Design review of the part built by this model. Coordinates are the model's own, in mm. A direction names the side the tool comes from. Give positions to 0.01 mm unless a question says otherwise; leave off trailing zeros. Loops run counter-clockwise (first coordinate to the right, second up) from the corner with the lowest first, then second, coordinate; pieces in that order, holes last. Notation, with made-up numbers: M 1.25,4.5 L 41.25,4.5 A29 cw 41.25,34.5 Z; hole C 47.5,38 d10. An arc over 180 degrees is marked long. Answer as CSV lines item,"result".
```python
from build123d import *

# Parameters (mm, degrees)
BOSS_EXTRUDE1_DEPTH = 8


with BuildPart() as part:
    # Sketch1 → Boss-Extrude1 (new body)
    with BuildSketch(Plane.XY):
        with BuildLine():
            Line((79.487889635, 127.207214423), (0, 0))
            Line((0, 0), (38, 0))
            ThreePointArc((38, 0), (40.636038969, 6.363961031), (47, 9))
            Line((47, 9), (99, 9))
            ThreePointArc((99, 9), (105.363961031, 6.363961031), (108, 0))
            Line((108, 0), (142, 0))
            Line((142, 0), (172.50354814, 93.880267937))
            ThreePointArc((172.50354814, 93.880267937), (166.569139078, 124.354715336), (137.573015724, 135.451290736))
            Line((137.573015724, 135.451290736), (79.487889635, 127.207214423))
        make_face()
        with BuildLine():
            ThreePointArc((130.852326035, 79.986711388), (131.785075785, 80.179945877), (132.735423682, 80.244757424))
            ThreePointArc((132.735423682, 80.244757424), (139.670612135, 74.195105322), (134.61852133, 66.50280346))
            ThreePointArc((134.61852133, 66.50280346), (133.68577158, 66.309568971), (132.735423682, 66.244757424))
            Line((132.735423682, 66.244757424), (99.049026675, 61.628618036))
            ThreePointArc((99.049026675, 61.628618036), (95.608426443, 60.298814317), (93.130184546, 57.566704329))
            ThreePointArc((93.130184546, 57.566704329), (61.402056741, 63.469750476), (90.372565984, 77.690497362))
            ThreePointArc((90.372565984, 77.690497362), (93.494426366, 75.725784751), (97.165929028, 75.370572))
            Line((97.165929028, 75.370572), (130.852326035, 79.986711388))
        make_face(mode=Mode.SUBTRACT)
    extrude(amount=BOSS_EXTRUDE1_DEPTH)


solid = part.part
```
1. We need section D-D, the plane x = 155. Write out the cut boundary in (y, z).
Answer block:
outline,"M 40.01,0 L 133.04,0 L 133.04,8 L 40.01,8 Z"
2. We need section C-C, the plane x = 68. Write out the cut boundary in (y, z).
Answer block:
outline,"M 9,0 L 52.21,0 L 52.21,8 L 9,8 Z; M 79.34,0 L 108.82,0 L 108.82,8 L 79.34,8 Z"
3. We need section B-B, the plane y = 52. Write out the cut boundary in (x, z), plus the area to 3 significant figures.
Answer block:
outline,"M 32.49,0 L 68.29,0 L 68.29,8 L 32.49,8 Z; M 88.2,0 L 158.9,0 L 158.9,8 L 88.2,8 Z"
area,"852 mm²"
4. For P1, Ø2, axis at y = 51, z = 2.5, coming from the +X side; P2, Ø1.5, axis at y = 19, z = 2, coming from the +X side; P3, Ø2, axis at y = 119.5, z = 4.5, coming from the +X side, all flat-tipped, find the tip position at first contact; note any pin that passes through.
Answer block:
P1,"x = 158.9"
P2,"x = 148.42"
P3,"x = 170.48"
5. For faces 1 (the cylindrical face through (105.294, 6.434, 3.944)), 2 (the cylindrical face through (95.651, 60.328, 3.944)), 3 (the flat face through (19, 0, 4)), list the 3-axis set-ups (+Z, -Z, +X, -X, +Y, -Y) from which the entire face can be reached by the end or side of a thin tool; tool diameter is ignored.
Answer block:
face 1,"+Z, -Z, -Y"
face 2,"+Z, -Z"
face 3,"+Z, -Z, +X, -X, -Y"
6. To check wall thickness, follow L1, parallel to Y at x = 77.5, z = 2; L2, parallel to X at y = 56.5, z = 3.5; L3, parallel to X at y = 58.5, z = 5.5. State the ranges of each line that lie inside material, in increasing order. Write a range as [from, to].
Answer block:
L1,"[9, 48.79], [82.76, 124.03]"
L2,"[35.31, 64], [92.49, 160.36]"
L3,"[36.55, 62.88], [93.73, 161.01]"
7. The part is to be moulded in two halves that separate along Y. For faces 4 (the flat face through (116.13, 63.97, 3.94)), 5 (the flat face through (105, 54, 0)), 6 (the flat face through (108.937, 131.387, 3.944)), say which applies: pulls with the +Y half, pulls with the -Y half, needs draft (parallel to the pull), parting line crosses it, or undercut.
Answer block:
face 4,"undercut"
face 5,"needs draft"
face 6,"pulls with the +Y half"
8. We need section A-A, the plane z = 2. Write out the cut boundary in (x, y), plus the area to 3 significant figures.
Answer block:
outline,"M 0,0 L 38,0 A9 cw 47,9 L 99,9 A9 cw 108,0 L 142,0 L 172.5,93.88 A32 ccw 137.57,135.45 L 79.49,127.21 Z; hole M 90.37,77.69 A17 ccw long 93.13,57.57 A8 cw 99.05,61.63 L 132.74,66.24 A7 ccw long 130.85,79.99 L 97.17,75.37 A8 cw Z"
area,"13,700 mm²"
